Build history of the part. All positions in model axes, mm. A direction names the side the tool comes from. Give positions to 0.01 mm unless a question says otherwise; leave off trailing zeros. Order: outer loops, then holes, each group sorted by start corner. A loop starts at its lowest first (then second) coordinate and runs counter-clockwise, first axis right, second up. Notation, with made-up numbers: (0.5, 63.5) - (5.5, 63.5) arc R16 ccw to (5.5, 87.5) - close; hole circle Ø11 at (67.5, 14.25). An arc over 180 degrees is marked (long way). One line per item, written item: value.
```python
from build123d import *

# Parameters (mm, degrees)
SKETCH1_W                                           = 196
SKETCH1_H                                           = 96
EXTRUDE1_DEPTH                                      = 17
CBORE_FOR_14_MM_LOCATING_GUIDE_BUSHING1_D           = 18
CBORE_FOR_14_MM_LOCATING_GUIDE_BUSHING1_CBORE_D     = 22
CBORE_FOR_14_MM_LOCATING_GUIDE_BUSHING1_CBORE_DEPTH = 6.1


with BuildPart() as part:
    # Sketch1 → Extrude1 (new body)
    with BuildSketch(Plane.XY):
        Rectangle(SKETCH1_W, SKETCH1_H)
    extrude(amount=-EXTRUDE1_DEPTH)

    # CBORE for 14 mm Locating Guide Bushing1 (through all)
    with Locations(Plane(origin=(49.246098405, -1.095802974, 0), x_dir=(-1, 0, 0), z_dir=(0, 0, 1))):
        with Locations((-10.753901595, -31.095802974), (109.246098405, -31.095802974), (109.246098405, 28.904197026), (-10.753901595, 28.904197026)):
            CounterBoreHole(CBORE_FOR_14_MM_LOCATING_GUIDE_BUSHING1_D / 2, CBORE_FOR_14_MM_LOCATING_GUIDE_BUSHING1_CBORE_D / 2, CBORE_FOR_14_MM_LOCATING_GUIDE_BUSHING1_CBORE_DEPTH)


solid = part.part
```
(1) Drill centre lines: line 1 (Y direction, x = -60, z = -4); line 2 (X direction, y = 35, z = -4.5); line 3 (X direction, y = -34, z = -14.25). Where is each one in solid material? Low to high.
Completed:
line 1: -48 to -41, -19 to 19, 41 to 48
line 2: -98 to -69.8, -50.2 to 50.2, 69.8 to 98
line 3: -98 to -68.06, -51.94 to 51.94, 68.06 to 98
(2) 3-axis set-ups, long thin cutter, end or side, ignore diameter. For faces 1 (the face through (58, 39, -6.1)), 2 (the face through (-51.416, -32.703, -11.626)): which of +Z, -Z, +X, -X, +Y, -Y reach the whole face in a straight line?
Completed:
face 1: +Z
face 2: +Z, -Z
(3) Slice it at A-A, the plane x = 60. Give the cut face in (y, z), and give its area (3 significant figures).
Completed:
outline: (-48, -17) - (-39, -17) - (-39, -6.1) - (-41, -6.1) - (-41, 0) - (-48, 0) - close; (-21, -17) - (21, -17) - (21, -6.1) - (19, -6.1) - (19, 0) - (-19, 0) - (-19, -6.1) - (-21, -6.1) - close; (39, -17) - (48, -17) - (48, 0) - (41, 0) - (41, -6.1) - (39, -6.1) - close
area: 971 mm²
(4) Pin check, flat tip, straight feed: P1, Ø20.5, axis at x = -60, y = 30, coming from the +Z side. Stop position of the tip, or through.
Completed:
P1: z = -6.1
(5) Slice it at D-D, the plane z = -3.25. Give the cut face in (x, y), and give its area (3 significant figures).
Completed:
outline: (-98, -48) - (98, -48) - (98, 48) - (-98, 48) - close; hole circle Ø22 at (-60, -30); hole circle Ø22 at (-60, 30); hole circle Ø22 at (60, -30); hole circle Ø22 at (60, 30)
area: 17,300 mm²
(6) Pull direction X, two halves, no side cores. Call faces 3 (the face through (-1, 1, -17)), 4 (the face through (98, -1, -8)), 5 (the face through (68.73, 36.69, -3.01)), 6 (the face through (-98, -1, -8)): +X half, -X half, draft (parallel to the pull), parting line (faces both ways), or undercut.
Completed:
face 3: draft
face 4: +X half
face 5: undercut
face 6: -X half
(7) Slice it at B-B, the plane y = 30. Give the cut face in (x, z), and give its area (3 significant figures).
Completed:
outline: (-98, -17) - (-69, -17) - (-69, -6.1) - (-71, -6.1) - (-71, 0) - (-98, 0) - close; (-51, -17) - (51, -17) - (51, -6.1) - (49, -6.1) - (49, 0) - (-49, 0) - (-49, -6.1) - (-51, -6.1) - close; (69, -17) - (98, -17) - (98, 0) - (71, 0) - (71, -6.1) - (69, -6.1) - close
area: 2,670 mm²
(8) Slice it at C-C, the plane z = -14.5. Give the cut face in (x, y), and give its area (3 significant figures).
Completed:
outline: (-98, -48) - (98, -48) - (98, 48) - (-98, 48) - close; hole circle Ø18 at (-60, -30); hole circle Ø18 at (-60, 30); hole circle Ø18 at (60, -30); hole circle Ø18 at (60, 30)
area: 17,800 mm²
